Autodesk Inventor part; units mm, degrees
ref_plane "ANBAU_XY" through (0, 0, -8.45) normal (0, 0, 1) x (1, 0, 0)
ref_plane "ANBAU_YZ" through (0, 0, -8.45) normal (1, 0, 0) x (0, 1, 0)
ref_plane "ANBAU_ZX" through (0, 0, -8.45) normal (0, 1, 0) x (0, 0, 1)
sketch "Sketch_1" plane through (0, 0, 0) normal (1, 0, 0) x (0, 1, 0)
  line L0 (0, -6.6953) -> (0, 0)
  line L1 (0, 0) -> (21.4, 0)
  line L2 (21.4, 0) -> (22, -0.6)
  line L3 (22, -0.6) -> (22, -7.85)
  line L4 (22, -7.85) -> (21.4, -8.45)
  line L5 (21.4, -8.45) -> (15.6, -8.45)
  arc A0 (15.6, -8.45) -> (15, -9.05) centre (15.6, -9.05) ccw
  line L6 (15, -9.05) -> (15, -44)
  line L7 (15, -44) -> (14, -45)
  line L8 (14, -45) -> (10, -45)
  line L9 (10, -45) -> (9.188, -44.188)
  line L10 (9.188, -44.188) -> (9.188, -12)
  line L11 (9.188, -12) -> (0, -6.6953)
  line L12 (0, -6.6953) -> (0, 0)
revolve "Revolution1" add sketch "Sketch_1" angle 360 about axis through (0, 0, -6.6953) along (0, 0, -1)
thread "Thread1"
sketch "Sketch_4" plane through (0, 0, -45) normal (0, 0, 1) x (1, 0, 0)
  line L0 (-18.5, -27) -> (18.5, -27)
  line L1 (18.5, -27) -> (18.5, 22)
  line L2 (18.5, 22) -> (13.5, 22)
  line L3 (13.5, 22) -> (13.5, -22)
  line L4 (13.5, -22) -> (-13.5, -22)
  line L5 (-13.5, -22) -> (-13.5, 22)
  line L6 (-13.5, 22) -> (-18.5, 22)
  line L7 (-18.5, 22) -> (-18.5, -27)
extrude "Extrusion1" cut sketch "Sketch_4" along normal blind 12
ref_plane "ANBAU_XY" through (0, 0, -8.45) normal (0, 0, 1) x (1, 0, 0)
ref_plane "ANBAU_YZ" through (0, 0, -8.45) normal (1, 0, 0) x (0, 1, 0)
ref_plane "ANBAU_ZX" through (0, 0, -8.45) normal (0, 1, 0) x (0, 0, 1)
ref_plane "EP_IP_XY" through (0, 0, 0) normal (0, 0, -1) x (1, 0, 0)
ref_plane "EP_IP_YZ" through (0, 0, 0) normal (1, 0, 0) x (0, -1, 0)
ref_plane "EP_IP_ZX" through (0, 0, 0) normal (0, -1, 0) x (0, 0, -1)
properties part number "1559400 EAGF-V2-KF-80/100---(GS)"
Geometry check sheet. Reference: the model listing, model coordinates, mm. A direction names the side the tool comes from. Round coordinates to 2 decimals unless told otherwise and drop trailing zeros. Loops run counter-clockwise (first coordinate to the right, second up) from the corner with the lowest first, then second, coordinate; pieces in that order, holes last. Notation, with made-up numbers: (80.5, 31.5) -> (96.5, 31.5) arc R34 ccw to (96.5, 68.5) -> close; hole circle Ø9 at (59, 8). An arc over 180 degrees is marked (long way). Use a Markdown table: item, result.
(1) Mould release check, pull along Y, two halves, no side actions. Record for faces 1 (the flat face through (3, -10, -45)), 2 (the cylindrical face through (-2.76, 8.764, -27.869)), 3 (the conical face through (-0.26, -14.17, -44.83)): released by +Y, released by -Y, zero draft, split by the parting line, or undercut.
Calculated:
| item | result |
|---|---|
| face 1 | zero draft |
| face 2 | undercut |
| face 3 | released by -Y |
(2) Go/stop test with flat-tipped pins: P1, Ø13, axis at y = 1, z = -41.5, coming from the +X side; P2, Ø8, axis at y = 12, z = -18.5, coming from the -X side; P3, Ø6, axis at y = -8.5, z = -9, coming from the -X side. Record where each tip stops, or that it passes through.
Calculated:
| item | result |
|---|---|
| P1 | x = 13.5 |
| P2 | x = -12.69 |
| P3 | x = -21.24 |
(3) Sectioned sample at A-A (z = -34). Enter the section's corners in (x, y).
Calculated:
| item | result |
|---|---|
| outline | (-13.5, -6.54) arc R15 ccw to (13.5, -6.54) -> (13.5, 6.54) arc R15 ccw to (-13.5, 6.54) -> close; hole circle Ø18.38 at (0, 0) |
(4) Sectioned sample at B-B (z = -18.5). Enter the section's corners in (x, y).
Calculated:
| item | result |
|---|---|
| outline | circle Ø30 at (0, 0); hole circle Ø18.38 at (0, 0) |
(5) Set-up check for faces 4 (the flat face through (14, 0, -33)), 5 (the cylindrical face through (-21.477, -4.769, -4.276)), 6 (the flat face through (-14, 0, -33)), 7 (the cylindrical face through (4.506, 14.307, -26.77)): record each of +Z, -Z, +X, -X, +Y, -Y from which the full face is reachable in a straight line by a thin tool's end or side.
Calculated:
| item | result |
|---|---|
| face 4 | -Z, +X, +Y, -Y |
| face 5 | +Z, -Z |
| face 6 | -Z, -X, +Y, -Y |
| face 7 | -Z |
(6) Scan lines: probe 1 along X at (y, z) = (0, -21); probe 2 along X at (y, z) = (0, -37); probe 3 along Y at (x, z) = (-8.5, -27). Record each from-to range of solid material in increasing order.
Calculated:
| item | result |
|---|---|
| probe 1 | -15 to -9.19, 9.19 to 15 |
| probe 2 | -13.5 to -9.19, 9.19 to 13.5 |
| probe 3 | -12.36 to -3.49, 3.49 to 12.36 |
